Check sheet for the modelled part. Datum: model origin and axes. Units: mm. Round coordinates to 2 decimals unless told otherwise and drop trailing zeros. Order: outer loops, then holes, each group sorted by start corner. A loop starts at its lowest first (then second) coordinate and runs counter-clockwise, first axis right, second up.
Q1. Cross-section at A-A on z = 23. Record the cut outline in (x, y), then the cut area to 3 significant figures.
Q2. Scan lines: probe 1 along X at (y, z) = (3749.5, 17.5); probe 2 along Y at (x, z) = (-288, 72); probe 3 along Y at (x, z) = (-835, 17). Record each from-to range of solid material in increasing order.
Q3. Cross-section at C-C on x = -398.5. Record the cut outline in (y, z), then the cut area to 3 significant figures.
Q4. Cross-section at B-B on y = 3836. Record the cut outline in (x, z).
Q5. Depth check by flat-ended pin: P1, Ø2, axis at x = -368.5, z = 39.5, coming from the +Y side; P2, Ø12, axis at x = -611, y = 3954, coming from the -Z side; P3, Ø1, axis at x = -566, z = 63.5, coming from the +Y side; P4, Ø3, axis at x = -467, z = 52, coming from the +Y side. Enter the tip coordinate at first touch or a pass-through.
Autodesk Inventor part; units mm, degrees
ref_plane "YZ Plane" through (0, 0, 0) normal (1, 0, 0) x (0, 1, 0)
ref_plane "XZ Plane" through (0, 0, 0) normal (0, 1, 0) x (-1, 0, 0)
ref_plane "XY Plane" through (0, 0, 0) normal (0, 0, 1) x (1, 0, 0)
sketch "Sketch1" plane through (0, 0, 0) normal (0, 0, 1) x (1, 0, 0)
  line L0 (-419.0894, 3166.7598) -> (-168.8434, 3166.7598)
  line L1 (-419.0894, 4266.7805) -> (-419.0894, 3166.7598)
  arc A0 (-419.0894, 4266.7805) -> (-968.8434, 3909.8415) centre (4748.6891, -4294.4149) ccw
  line L2 (-968.8434, 2366.6217) -> (-968.8434, 3909.8415)
  line L3 (-168.8434, 2366.6217) -> (-968.8434, 2366.6217)
  line L4 (-168.8434, 3166.7598) -> (-168.8434, 2366.6217)
extrude "Extrusion1" add sketch "Sketch1" along normal blind 80
properties part number "front_wall_block03" material "Wood (Maple)"
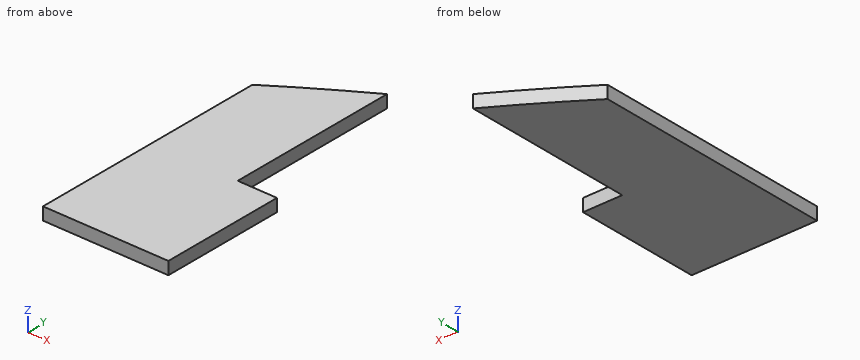
Results found:
1. outline: (-968.84, 2366.62) - (-168.84, 2366.62) - (-168.84, 3166.76) - (-419.09, 3166.76) - (-419.09, 4266.78) arc R9999.98 ccw to (-968.84, 3909.84) - close
1. area: 1,150,000 mm2
2. probe 1: x = -968.84 to -419.09
2. probe 2: y = 2366.62 to 3166.76
2. probe 3: y = 2366.62 to 4001.51
3. outline: (2366.62, 0) - (3166.76, 0) - (3166.76, 80) - (2366.62, 80) - close
3. area: 64,000 mm2
4. outline: (-968.84, 0) - (-419.09, 0) - (-419.09, 80) - (-968.84, 80) - close
5. P1: stops at y = 3166.76
5. P2: stops at z = 0
5. P3: stops at y = 4176.68
5. P4: stops at y = 4238.59
